Read the model definition and answer for the solid it produces. Units are mm, in the model's axes. Give positions to 0.01 mm unless a question says otherwise; leave off trailing zeros. Write item = value, one per line.
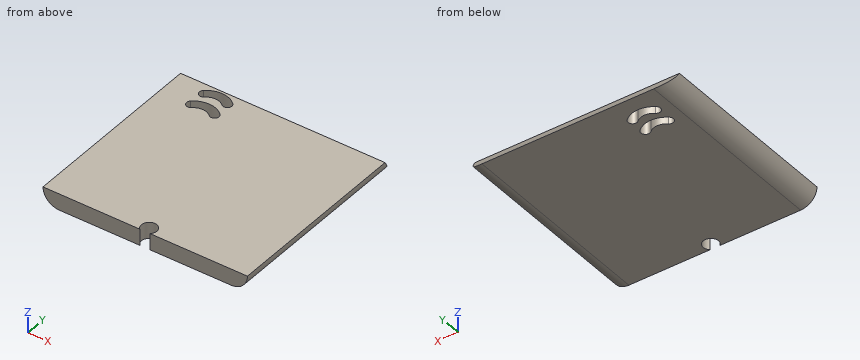
Autodesk Inventor part; units mm, degrees
ref_plane "YZ Plane" through (0, 0, 0) normal (1, 0, 0) x (0, 1, 0)
ref_plane "XZ Plane" through (0, 0, 0) normal (0, 1, 0) x (-1, 0, 0)
ref_plane "XY Plane" through (0, 0, 0) normal (0, 0, 1) x (1, 0, 0)
sketch "Sketch2" plane through (0, 0, 0) normal (1, 0, 0) x (0, 1, 0)
  line L0 (43.74, 0) -> (-43.74, 0) construction
  line L1 (0, 65.172) -> (0, -65.172) construction
  spline S0 degree 3 poles (-5.8666, 35) (13.8832, 21.2522) (-10.0462, -16.0043) (8.551, -35) knots 1 1 1 1 2 2 2 2
  line L2 (-5.8666, 35) -> (13.8832, 21.2522) construction
  line L3 (13.8832, 21.2522) -> (-10.0462, -16.0043) construction
  line L4 (-10.0462, -16.0043) -> (8.551, -35) construction
  line L5 (-5.8666, 35) -> (-40.8666, 35)
  line L6 (-1.7165, 31) -> (-40.8666, 31)
  line L7 (-40.8666, 35) -> (-40.8666, 31)
  line L8 (8.551, -35) -> (-40.8666, -35)
  line L9 (-40.8666, -35) -> (-40.8666, -31)
  line L10 (-40.8666, -31) -> (5.392, -31)
  point P0 (0, 0)
  point P1 (0, 0)
  point P2 (0, 0)
  point P3 (0, 0)
  point P4 (0, 0)
  dimension "d0" = 35
  dimension "d1" = 4
  dimension "d2" = 4
extrude "Extrusion1" add sketch "Sketch2" along normal blind 50 contours S0 L8 L9 L10
fillet "Fillet1" radius 4 2 edges at (50, -16.1578, -35) (0, -16.1578, -35)
sketch "Sketch3" plane through (46, 8.551, -35) normal (0, 0, -1) x (-1, 0, 0)
  circle A0 centre (21.067, -48.0176) radius 1.875
  line L0 (42, -49.4176) -> (0, -49.4176)
  arc A1 (38.2925, -5.9026) -> (32.5085, -5.9701) centre (35.4376, -9.1181) ccw construction
  arc A2 (39.0228, -5.08) -> (31.7591, -5.1648) centre (35.4376, -9.1181) ccw
  arc A3 (37.5622, -6.7252) -> (33.2578, -6.7754) centre (35.4376, -9.1181) ccw
  arc A4 (37.5622, -6.7252) -> (39.0228, -5.08) centre (38.2925, -5.9026) ccw
  arc A5 (31.7591, -5.1648) -> (33.2578, -6.7754) centre (32.5085, -5.9701) ccw
  arc A6 (38.2925, -10.2026) -> (32.5085, -10.2701) centre (35.4376, -13.4181) ccw construction
  arc A7 (39.0228, -9.38) -> (31.7591, -9.4648) centre (35.4376, -13.4181) ccw
  arc A8 (37.5622, -11.0252) -> (33.2578, -11.0754) centre (35.4376, -13.4181) ccw
  arc A9 (37.5622, -11.0252) -> (39.0228, -9.38) centre (38.2925, -10.2026) ccw
  arc A10 (31.7591, -9.4648) -> (33.2578, -11.0754) centre (32.5085, -10.2701) ccw
  line L1 (35.4376, -14.6833) -> (35.4376, -1.9908) construction
  point P0 (46, -8.551)
  dimension "d6" = 3.75
  dimension "d7" = 1.4
  dimension "d10" = 4.3
  dimension "d11" = 4.3
  dimension "d12" = 3.2
  dimension "d13" = 3.2
  dimension "d14" = 4.3
extrude "Extrusion2" cut sketch "Sketch3" against normal blind 4
equation "\"d11\" = d10"
equation "\"d13\" = d12"
equation "\"d14\" = d11"
properties part number "Case Back"
1. Section B-B (x = 9.5) is taken. Count the separate pieces of the cut face and the enclosed holes in it, and give its area (3 significant figures).
Recorded:
separate_pieces = 3
enclosed_holes = 0
area = 173 mm^2
2. Straight lines are drawn through the part: L1, parallel to Y at x = 10.5, z = -33.4; L2, parallel to Y at x = 12.5, z = -33.5; L3, parallel to X at y = -38, z = -31.7. For each, find the intervals that lie inside material, in ascending order. Write a range as [from, to].
Recorded:
L1 = [-40.87, -1.67], [0.53, 2.63], [4.83, 7.12]
L2 = [-40.87, -2.32], [0.17, 1.98], [4.47, 7.2]
L3 = [0.06, 23.76], [26.1, 49.94]
3. Flat-ended cylindrical pins translate along their axes: pin 1 (1.5 mm diameter, centred on x = 27.5, z = -33, fed in from +Y); pin 2 (1 mm diameter, centred on y = -24.5, z = -32.5, fed in from -X); pin 3 (2 mm diameter, centred on x = 24.93, y = -39.47, fed in from +Z). Find the tip coordinate at first contact, or state that the pin passes through.
Recorded:
pin_1 = 7.41
pin_2 = 0.13
pin_3 = through
